Autodesk Inventor part; units mm, degrees
ref_plane "Plano de trabajo1" through (0, -10, 0) normal (0, -1, 0) x (1, 0, 0)
ref_plane "YZ Plane" through (0, 0, 0) normal (1, 0, 0) x (0, 1, 0)
ref_plane "XZ Plane" through (0, 0, 0) normal (0, 1, 0) x (-1, 0, 0)
sketch "Boceto1" plane through (0, 0, 0) normal (0, 1, 0) x (-1, 0, 0)
  line L0 (0, 0) -> (-4, 0)
  line L1 (-4, 0) -> (-4, -9.5)
  line L2 (-4, -9.5) -> (0, -9.5)
  line L3 (0, -9.5) -> (0, 0)
  dimension "d0" = 4
  dimension "d1" = 9.5
extrude "Extrusión1" add sketch "Boceto1" along normal blind 4
sketch "Boceto2" plane through (0, 0, -9.5) normal (-1, 0, 0) x (0, 0, 1)
  line L0 (9.5, 4) -> (0, 4)
  line L1 (9.5, 4) -> (-4.5, 4)
  line L2 (-4.5, 4) -> (-7.5, 4)
  line L3 (-5, 0) -> (-5, -16)
  line L4 (0, 0) -> (0, 4)
  line L5 (9.5, 0) -> (0, 0)
  line L6 (0, 0) -> (9.5, 0)
  line L7 (9.5, 0) -> (9.5, 4)
  line L8 (-5, -16) -> (-12.5, -16)
  line L9 (-12.5, -16) -> (-12.5, 4)
  line L10 (-12.5, 4) -> (-7.5, 4)
  line L11 (-5, 0) -> (9.5, 0)
  line L12 (-5, 4) -> (9.5, 4)
  line L13 (9.5, 0) -> (9.5, 4)
  line L14 (9.5, 0) -> (9.5, 4)
  dimension "d4" = 14
  dimension "d5" = 3
  dimension "d6" = 20
  dimension "d25" = 7.5
extrude "Extrusión2" add sketch "Boceto2" along normal blind 2 contours L7 L5 L4 L0
sketch "Boceto3" plane through (-2, 0, -9.5) normal (-1, 0, 0) x (0, 0, 1)
  line L0 (9.5, 4) -> (0, 4)
  line L1 (-7.5, 4) -> (-2.5, 4)
  line L2 (-2.5, 4) -> (-2.5, 1.5)
  line L3 (-2.5, 1.5) -> (-7.5, 1.5)
  line L4 (-7.5, 4) -> (-7.5, -16)
  line L5 (-7.5, 1.5) -> (-7.5, -4.5)
  line L6 (-7.5, -4.5) -> (-7.5, -10.5)
  line L7 (-7.5, -10.5) -> (-7.5, -13)
  line L8 (-7.5, -13) -> (-2.5, -13)
  line L9 (-2.5, -13) -> (-2.5, -10.5)
  line L10 (-2.5, -10.5) -> (-7.5, -10.5)
  line L11 (-7.5, -4.5) -> (-7.5, -5.75)
  line L12 (-7.5, -5.75) -> (-2.5, -5.75)
  line L13 (-2.5, -5.75) -> (-2.5, -3.25)
  line L14 (-2.5, -3.25) -> (-7.5, -3.25)
  point P0 (9.5, 0)
  dimension "d9" = 5
  dimension "d10" = 2.5
  dimension "d11" = 6
  dimension "d12" = 6
  dimension "d13" = 2.5
  dimension "d14" = 5
  dimension "d15" = 2.5
  dimension "d16" = 1.25
  dimension "d17" = 5
  dimension "d18" = 2.5
extrude "Extrusión3" cut sketch "Boceto3" against normal blind 1
chamfer "Chaflán1" distance 2 angle 45 2 edges at (4, 2, -9.5) (4, 2, 0)
sketch "Boceto4" plane through (-2, 0, -9.5) normal (-1, 0, 0) x (0, 0, 1)
  line L0 (0, 0) -> (9.5, 0)
  line L1 (9.5, 0) -> (0, 0)
  line L2 (0, 0) -> (-5, 0)
  line L3 (-5, 0) -> (-5, -20)
  line L4 (-5, -20) -> (-12.5, -20)
  line L5 (-12.5, -20) -> (-12.5, 4)
  line L6 (9.5, 4) -> (0, 4)
  line L7 (-12.5, 4) -> (9.5, 4)
  line L8 (9.5, 0) -> (9.5, 4)
  line L9 (9.5, 4) -> (9.5, 0)
  line L10 (-12.5, 4) -> (-7.5, 4)
  line L11 (-7.5, 4) -> (-7.5, 1.5)
  line L12 (-7.5, 1.5) -> (-12.5, 1.5)
  line L13 (-12.5, 1.2493) -> (-12.5, -4.7507)
  line L14 (-12.5, -4.7507) -> (-12.5, -10.7507)
  line L15 (-12.5, -10.7507) -> (-7.5, -10.7507)
  line L16 (-7.5, -10.7507) -> (-7.5, -13.2507)
  line L17 (-7.5, -13.2507) -> (-12.5, -13.2507)
  line L18 (-12.5, -4.7507) -> (-12.5, -6.0007)
  line L19 (-12.5, -6.0007) -> (-7.5, -6.0007)
  line L20 (-7.5, -6.0007) -> (-7.5, -3.5007)
  line L21 (-7.5, -3.5007) -> (-12.5, -3.5007)
  dimension "d26" = 5
  dimension "d27" = 20
  dimension "d28" = 7.5
  dimension "d29" = 5
  dimension "d30" = 2.5
  dimension "d31" = 6
  dimension "d32" = 6
  dimension "d33" = 5
  dimension "d34" = 2.5
  dimension "d35" = 1.25
  dimension "d36" = 2.5
extrude "Extrusión4" add sketch "Boceto4" along normal blind 3 contours L2 L3 L4 L5 L17 L16 L15 L19 L20 L21 L12 L11 L7 L6 L8 L0
sketch "Boceto5" plane through (0, 4, 0) normal (0, 1, 0) x (1, 0, 0)
  line L0 (-2, 17) -> (-5, 17)
  line L1 (-5, 17) -> (-2, 17)
  line L2 (-2, 14.5) -> (-2, 9.5)
  line L3 (-2, 17) -> (-2, 9.5)
  line L4 (2, 9.5) -> (-2, 9.5)
  line L5 (-2, 9.5) -> (2, 9.5)
  line L6 (4, 7.5) -> (2, 9.5)
  line L7 (2, 9.5) -> (4, 7.5)
  line L8 (4, 2) -> (4, 7.5)
  line L9 (4, 7.5) -> (4, 2)
  line L10 (2, 0) -> (4, 2)
  line L11 (4, 2) -> (2, 0)
  line L12 (2, 0) -> (-5, 0)
  line L13 (2, 0) -> (-5, 0)
  line L14 (-5, 0) -> (-5, 17)
  line L15 (-5, 0) -> (-5, 17)
  point P0 (0, 0)
extrude "Extrusión5" add sketch "Boceto5" along normal blind 2.5
sketch "Boceto7" plane through (-5, 0, -9.5) normal (-1, 0, 0) x (0, 0, 1)
  line L0 (-7.5, 1.5) -> (-7.5, 6.5)
  line L1 (-7.5, 1.5) -> (-7.5, -20)
  line L2 (-12.5, -20) -> (-5, -20)
  line L3 (-7.5, -20) -> (-5.5, -20)
  line L4 (-5.5, -20) -> (-5.5, 6.5)
  line L5 (0, 6.5) -> (-7.5, 6.5)
  line L6 (-7.5, 6.5) -> (-7.5, 1.5)
  point P0 (9.5, 0)
  dimension "d41" = 2
extrude "Extrusión6" add sketch "Boceto7" along normal blind 8
sketch "Boceto8" plane through (-2, -13.2507, -17) normal (0, 0, -1) x (-1, 0, 0)
  line L0 (0, 14.7507) -> (0, 19.7507)
  line L1 (0, 14.7507) -> (2, 14.7507)
  line L2 (2, 14.7507) -> (6, 14.7507)
  line L3 (6, 14.7507) -> (6, 19.7507)
  line L4 (3, 19.7507) -> (11, 19.7507)
  circle A0 centre (6, 14.7507) radius 1
  line L5 (6, 13.7507) -> (6, 7.7507)
  line L6 (6, 7.7507) -> (6, 6.1507)
  circle A1 centre (6, 6.1507) radius 1
  line L7 (6, 6.1507) -> (5.7406, 6.1507)
  point P0 (-2, 13.2507)
  dimension "d46" = 2
  dimension "d44" = 2
  dimension "d45" = 4
  dimension "d47" = 6
extrude "Extrusión7" add sketch "Boceto8" along normal blind 6
sketch "Boceto9" plane through (-2, -20, -14.5) normal (0, 0, 1) x (1, 0, 0)
  line L0 (0, 0) -> (0, 20)
  line L1 (0, 20) -> (-3, 20)
  line L2 (0, 20) -> (-3, 20)
  line L3 (-3, 0) -> (-11, 0)
  line L4 (-3, 20) -> (-3, 0)
  line L5 (0, 0) -> (-3, 0)
  line L6 (-3, 0) -> (0, 0)
  line L7 (0, 0) -> (0, 20)
  point P0 (2, 20)
extrude "Extrusión8" cut sketch "Boceto9" against normal blind 0.5
sketch "Boceto10" plane through (-2, -3.5007, -22) normal (0, 0, -1) x (-1, 0, 0)
  line L0 (0, 5.0007) -> (3, 5.0007)
  line L1 (0, 5.0007) -> (0, 0)
  line L2 (3, 5.0007) -> (0, 5.0007)
  line L3 (0, 5.0007) -> (0, 0)
  line L4 (0, 0) -> (3, 0)
  line L5 (3, 0) -> (3, 5.0007)
  line L6 (0, -2.5) -> (3, -2.5)
  line L7 (0, -7.25) -> (3, -7.25)
  line L8 (3, -2.5) -> (0, -2.5)
  line L9 (0, -2.5) -> (0, -7.25)
  line L10 (0, -7.25) -> (3, -7.25)
  line L11 (3, -7.25) -> (3, -2.5)
  line L12 (3, -16.4993) -> (3, -9.75)
  line L13 (0, 3.5007) -> (0, -16.4993)
  line L14 (3, -9.75) -> (0, -9.75)
  line L15 (0, -9.75) -> (0, -16.4993)
  line L16 (0, -16.4993) -> (3, -16.4993)
  line L17 (3, -16.4993) -> (3, -9.75)
  point P0 (-2, 3.5007)
extrude "Extrusión9" cut sketch "Boceto10" against normal blind 5
sketch "Boceto11" plane through (-5, 0, -15) normal (0, 0, 1) x (1, 0, 0)
  line L0 (0, 0) -> (0, -20)
  point P0 (5, 0)
  dimension "d58" = 20
ref_plane "Plano de trabajo1" through (0, -10, 0) normal (0, -1, 0) x (1, 0, 0)
mirror "Simetría1" about plane through (0, -10, 0) normal (0, -1, 0) of "Extrusión5"
sketch "Boceto12" plane through (-5, -24, 0) normal (0, 1, 0) x (1, 0, 0)
  line L0 (0, 0) -> (7, 0)
  line L1 (0, 17) -> (0, 0)
  line L2 (0, 0) -> (0, 17)
  line L3 (3, 9.5) -> (3, 17)
  line L4 (0, 17) -> (3, 17)
  line L5 (3, 17) -> (3, 9.5)
  line L6 (7, 9.5) -> (3, 9.5)
  line L7 (3, 9.5) -> (7, 9.5)
  line L8 (9, 7.5) -> (7, 9.5)
  line L9 (7, 9.5) -> (9, 7.5)
  line L10 (9, 2) -> (9, 7.5)
  line L11 (9, 7.5) -> (9, 2)
  line L12 (9, 2) -> (7, 0)
  line L13 (7, 0) -> (0, 0)
  point P0 (5, 0)
extrude "Extrusión10" add sketch "Boceto12" along normal blind 4
sketch "Boceto13" plane through (0, 6.5, 0) normal (0, 1, 0) x (1, 0, 0)
  line L0 (-5, 15) -> (-2, 15)
  line L1 (-5, 15) -> (10.3969, 15)
  line L2 (10.3969, 15) -> (10.0462, -8.8687)
  line L3 (10.0462, -8.8687) -> (-11.5494, -8.8687)
  line L4 (-11.5494, -8.8687) -> (-11.5494, 15)
  line L5 (-5, 15) -> (-13, 15)
  line L6 (-5, 15) -> (-11.5494, 15)
  point P0 (0, 0)
extrude "Extrusión11" cut sketch "Boceto13" against normal blind 9
sketch "Boceto14" plane through (-13, -20, -17) normal (0, -1, 0) x (1, 0, 0)
  line L0 (11, 0) -> (0, 0)
  line L1 (8, 2) -> (0, 2)
  line L2 (0, 0) -> (8, 0)
  line L3 (8, 0) -> (8, 2)
  line L4 (8, 2) -> (0, 2)
  line L5 (0, 2) -> (0, 0)
  point P0 (13, 17)
extrude "Extrusión12" add sketch "Boceto14" along normal blind 6.5
sketch "Boceto15" plane through (-2, 6.5, -17) normal (0, 0, -1) x (-1, 0, 0)
  line L0 (0, 0) -> (11, 0)
  line L1 (5.9919, 0) -> (15.9919, 0)
  line L2 (15.9919, 0) -> (15.9919, -33)
  circle A0 centre (6, -5) radius 1
  line L3 (6, -5) -> (25.1824, -5)
  circle A1 centre (6, -13.6) radius 1
  line L4 (6, -13.6) -> (25.934, -13.6)
  circle A2 centre (15.9919, -5) radius 1
  circle A3 centre (15.967, -13.6) radius 1
  line L5 (11, 0) -> (21, 0)
  line L6 (21, 0) -> (21, -33)
  line L7 (11, 0) -> (11, -33)
  line L8 (21, -33) -> (11, -33)
  line L9 (11, -33) -> (11, 0)
  point P0 (-2, -6.5)
  dimension "d66" = 10
  dimension "d67" = 2
  dimension "d68" = 2
  dimension "d69" = 10
extrude "Extrusión13" add sketch "Boceto15" against normal blind 2 contours L1 L2 A2 L3 L7 | L5 L6 L3 A2 L2 | L3 A2 L2 A3 L4 L7 | A2 L3 L2 | L2 L3 A2 | L3 L2 A2 | L4 A3 L2 L8 L7 | L3 A2 L2 | L3 L6 L4 A3 L2 A2 | A3 L2 L4 | L4 L2 A3 | L6 L8 L2 A3 L4 | A3 L4 L2 | L4 A3 L2
sketch "Boceto16" plane through (-2, -26.5, -17) normal (0, 0, -1) x (-1, 0, 0)
  circle A0 centre (6, 28) radius 1
  line L0 (6, 28) -> (16, 28)
  circle A1 centre (6, 19.4) radius 1
  line L1 (6, 19.4) -> (16, 19.4)
  circle A2 centre (16, 28) radius 1
  circle A3 centre (16, 19.4) radius 1
  point P0 (-2, 26.5)
  dimension "d72" = 10
  dimension "d73" = 10
  dimension "d74" = 2
  dimension "d75" = 2
extrude "Extrusión14" add sketch "Boceto16" along normal blind 6 contours A2 | A3
sketch "Boceto17" plane through (-8, -7.1, -23) normal (0, 0, -1) x (-1, 0, 0)
  line L0 (4.3511, -2.3199) -> (4.3511, 11.9603)
  line L1 (4.3511, 11.9603) -> (-3.8663, 11.9603)
  line L2 (-3.8663, 11.9603) -> (-3.8663, -2.9713)
  line L3 (-3.8663, -2.9713) -> (4.3511, -2.3199)
  point P0 (-8, 7.1)
extrude "Extrusión15" cut sketch "Boceto17" against normal blind 6
sketch "Boceto18" plane through (-2, -26.5, -17) normal (0, 0, -1) x (-1, 0, 0)
  line L0 (3, 6.5) -> (3, 0)
  line L1 (0, 0) -> (3, 0)
  line L2 (3, 0) -> (3, 33)
  line L3 (0, 33) -> (21, 33)
  line L4 (0, 33) -> (21, 33)
  line L5 (3, 33) -> (0, 33)
  line L6 (0, 33) -> (0, 0)
  line L7 (3, 0) -> (-4, 0)
  line L8 (-4, 0) -> (0, 0)
  line L9 (3, 0) -> (0, 0)
  line L10 (1.5, 33) -> (1.5, 0)
  line L11 (1.5, 33) -> (1.5, 23)
  circle A0 centre (1.5, 23) radius 1
  line L12 (1.5, 0) -> (1.5, 10)
  circle A1 centre (1.5, 10) radius 1
  point P0 (-2, 26.5)
  dimension "d82" = 10
  dimension "d83" = 2
  dimension "d84" = 10
  dimension "d85" = 2
extrude "Extrusión16" add sketch "Boceto18" along normal blind 5 contours L0 L1 L10 A1 A0 L3 L2 | L1 L6 L3 L10 A0 A1
sketch "Boceto19" plane through (-5, -20, -15) normal (0, 0, 1) x (1, 0, 0)
  line L0 (3, 0) -> (-18, 0)
  line L1 (-18, 26.5) -> (-18, -6.5)
  line L2 (-18, 0) -> (-18, 5)
  line L3 (-18, 5) -> (2.826, 5)
  line L4 (2.826, 5) -> (3, 5)
  line L5 (3, 26.5) -> (3, 0)
  line L6 (3, 5) -> (3, 0)
  point P0 (5, 20)
  dimension "d86" = 5
extrude "Extrusión17" add sketch "Boceto19" along normal blind 5
sketch "Boceto20" plane through (-23, -20, -15) normal (0, -1, 0) x (1, 0, 0)
  line L0 (0, 0) -> (0, 5)
  line L1 (0, 5) -> (18, 5)
  line L2 (0, 0) -> (18, 0)
  line L3 (18, 0) -> (18, 5)
  line L4 (18, 5) -> (0, 5)
  line L5 (0, 5) -> (0, 0)
  point P0 (23, 15)
extrude "Extrusión18" add sketch "Boceto20" along normal blind 6.5
sketch "Boceto21" plane through (-5, -26.5, -17) normal (-1, 0, 0) x (0, 0, 1)
  point P0 (17, 26.5)
properties part number "base_fin_carrera"
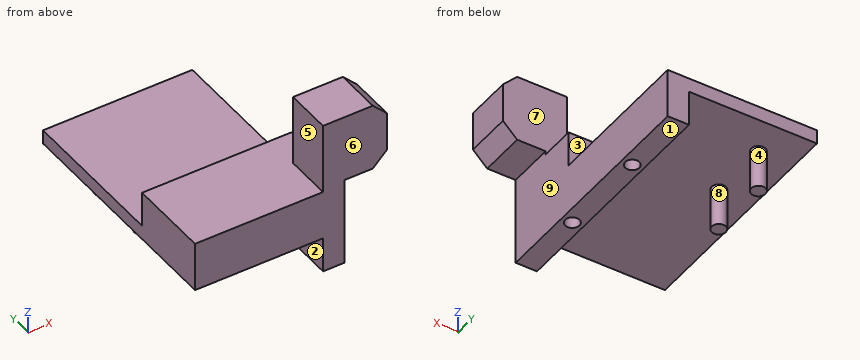
Source: CAD feature listing. Evaluate the final solid. Frame: model axes, mm. Face numbers are marked on the shaded views. A direction names the side the tool comes from. Round coordinates to 2 decimals unless told otherwise and drop trailing zeros. Loops run counter-clockwise (first coordinate to the right, second up) from the corner with the lowest first, then second, coordinate; pieces in that order, holes last. Notation, with made-up numbers: (80, -3.75) -> (135, -3.75) arc R14 cw to (135, 1.25) -> close; hole circle Ø4 at (68.5, 65). An arc over 180 degrees is marked (long way). Answer as a JSON object with one key per item and string values. Group by question number.
Q1. Section query D-D (y = -20.5). Output: boundary loops of the cut face in (x, z), plus the area to 3 significant figures.
Q2. Section query B-B (x = -18). Output: boundary loops of the cut face in (y, z), plus the area to 4 significant figures.
Q3. Access query for the marked faces 1, 2, 3, 4 and 5. Directions: +Z, -Z, +X, -X, +Y, -Y. A direction counts if a zero-diameter tool reaches every point of the face in a straight line with its end or side. Return the directions, or none.
Q4. Mould query, pull axis Y, two halves, no side actions, for the marked faces 6, 7, 8 and 9. Classes: pulls with the +Y half, pulls with the -Y half, needs draft (parallel to the pull), parting line crosses it, or undercut.
Q5. Section query C-C (z = -5.5). Output: boundary loops of the cut face in (x, y).
Q6. Ray query, line 1 (Y direction, x = -3.5, z = -20.85); line 2 (X direction, y = -3.5, z = -19.35); line 3 (Y direction, x = -3.5, z = -9). Return the intervals inside material, ascending. Write a range as from..to.
Q7. Contact query for flat-ended pins moving along their axis: P1, Ø1.6, axis at x = -3.5, y = -16.5, coming from the -Z side; P2, Ø8, axis at x = -19.5, y = -17, coming from the +Z side; P3, Ø6, axis at y = -18.5, z = -16.5, coming from the +X side. Output: stop coordinate, or through.
Q8. Section query A-A (y = -16.5). Output: boundary loops of the cut face in (x, z), plus the area to 3 significant figures.
Completed:
{
 "1": {"outline": "(-23, -17) -> (-5, -17) -> (-5, -22) -> (-2, -22) -> (-2, -9.5) -> (2, -9.5) -> (4, -7.5) -> (4, -2) -> (2, 0) -> (-5, 0) -> (-5, -10) -> (-23, -10) -> close", "area": "245 mm²"},
 "2": {"outline": "(-26.5, -17) -> (-8.1, -17) -> (-8.1, -23) -> (-6.1, -23) -> (-6.1, -17) -> (0.5, -17) -> (0.5, -23) -> (2.5, -23) -> (2.5, -17) -> (6.5, -17) -> (6.5, -15) -> (-15, -15) -> (-15, -10) -> (-26.5, -10) -> close", "area": "147.5 mm²"},
 "3": {"face 1": "-Z, +X, +Y, -Y", "face 2": "-Z, +Y, -Y", "face 3": "+Z, +X, -X, +Y", "face 4": "-Z", "face 5": "+Z, -X, +Y, -Y"},
 "4": {"face 6": "pulls with the -Y half", "face 7": "pulls with the +Y half", "face 8": "undercut", "face 9": "needs draft"},
 "5": {"outline": "(-5, -26.5) -> (4, -26.5) -> (4, -20) -> (-5, -20) -> close"},
 "6": {"line 1": "-26.5..-17.5, -15.5..-4.5, -2.5..6.5", "line 2": "-5..-4.5, -2.5..-2", "line 3": "-26.5..-20"},
 "7": {"P1": "z = -17", "P2": "z = -10", "P3": "x = -2"},
 "8": {"outline": "(-23, -17) -> (-5, -17) -> (-5, -22) -> (-4.5, -22) -> (-4.5, -17) -> (-2.5, -17) -> (-2.5, -22) -> (-2, -22) -> (-2, -10) -> (-23, -10) -> close", "area": "152 mm²"}
}
